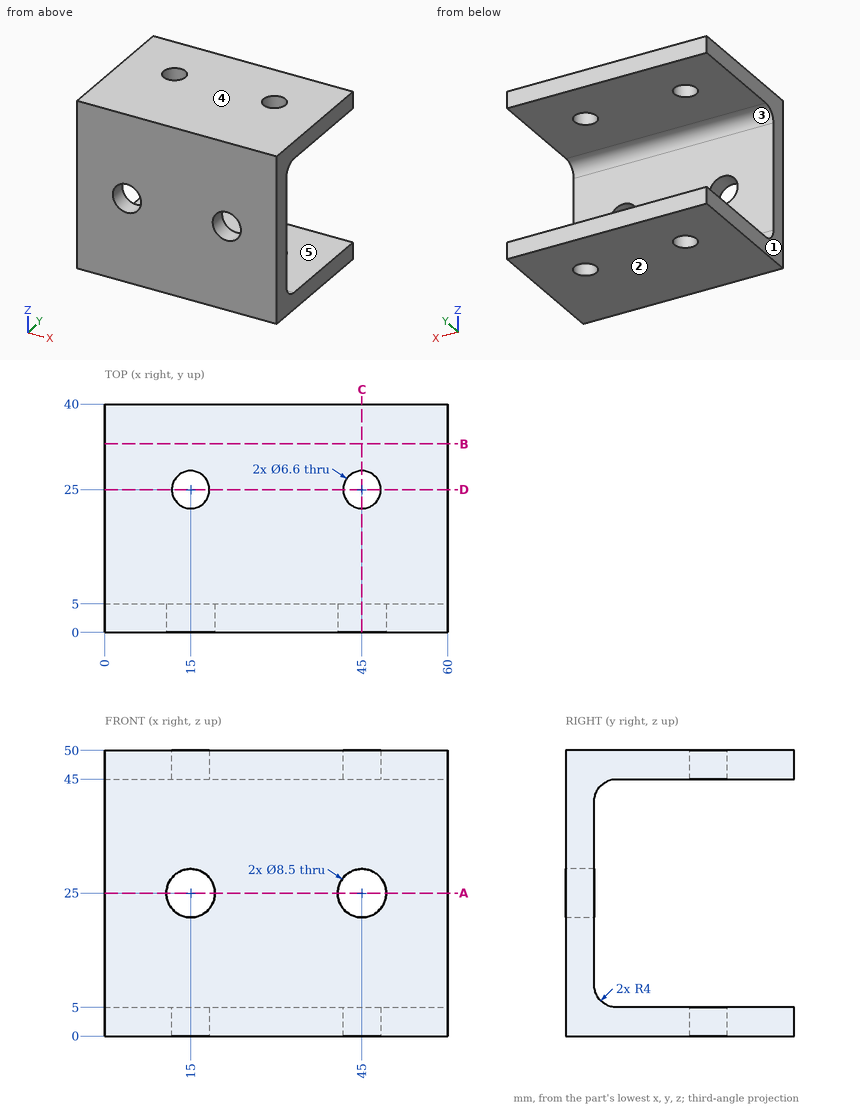
Here's the drawing with two shaded views (mm, measured from the low corner). I have some questions. A direction names the side the tool comes from. Give positions to 0.01 mm unless a question says otherwise; leave off trailing zeros. Order: outer loops, then holes, each group sorted by start corner. A loop starts at its lowest first (then second) coordinate and runs counter-clockwise, first axis right, second up. Notation, with made-up numbers: (70, 66.25) -> (109, 66.25) arc R19 ccw to (109, 90.25) -> close; hole circle Ø8 at (19, 22). An arc over 180 degrees is marked (long way). One line per item, written item: value. Start each with the question number.
1. Will these pins go through, and if not, where does the flat tip stop? pin 1 Ø1 at (x, y) = (51.5, 24) entering from -Z; pin 2 Ø1 at (x, z) = (47, 18) entering from +Y.
2. Imagine slicing it at D-D, the plane y = 25. List the corners of the cut face in (x, z) for me, plus the area to 3 significant figures.
3. Imagine slicing it at A-A, the plane z = 25. List the corners of the cut face in (x, y) for me.
4. Imagine slicing it at C-C, the plane x = 45. List the corners of the cut face in (y, z) for me, plus the area to 3 significant figures.
5. I need wall thicknesses on probe 1 along X at (y, z) = (1, 25); probe 2 along Z at (x, y) = (52.5, 24); probe 3 along Y at (x, z) = (15, 3). Which ranges of each line are inside material? Lowest first, please. Write a range as from..to.
6. Imagine slicing it at B-B, the plane y = 33. List the corners of the cut face in (x, z) for me, plus the area to 3 significant figures.
7. We'd pull the mould along Z, two halves only. Please class the marked faces 1, 2 and 3: released by +Z, released by -Z, zero draft, split by the parting line, or undercut.
8. For the marked faces 4 and 5, which set-ups out of +Z, -Z, +X, -X, +Y, -Y let a thin tool reach every point of the face, with its end or its side?
Values follow:
1. pin 1: stops at z = 0
1. pin 2: stops at y = 5
2. outline: (0, 0) -> (11.7, 0) -> (11.7, 5) -> (0, 5) -> close; (0, 45) -> (11.7, 45) -> (11.7, 50) -> (0, 50) -> close; (18.3, 0) -> (41.7, 0) -> (41.7, 5) -> (18.3, 5) -> close; (18.3, 45) -> (41.7, 45) -> (41.7, 50) -> (18.3, 50) -> close; (48.3, 0) -> (60, 0) -> (60, 5) -> (48.3, 5) -> close; (48.3, 45) -> (60, 45) -> (60, 50) -> (48.3, 50) -> close
2. area: 468 mm2
3. outline: (0, 0) -> (10.75, 0) -> (10.75, 5) -> (0, 5) -> close; (19.25, 0) -> (40.75, 0) -> (40.75, 5) -> (19.25, 5) -> close; (49.25, 0) -> (60, 0) -> (60, 5) -> (49.25, 5) -> close
4. outline: (0, 0) -> (21.7, 0) -> (21.7, 5) -> (9, 5) arc R4 cw to (5, 9) -> (5, 20.75) -> (0, 20.75) -> close; (0, 29.25) -> (5, 29.25) -> (5, 41) arc R4 cw to (9, 45) -> (21.7, 45) -> (21.7, 50) -> (0, 50) -> close; (28.3, 0) -> (40, 0) -> (40, 5) -> (28.3, 5) -> close; (28.3, 45) -> (40, 45) -> (40, 50) -> (28.3, 50) -> close
4. area: 498 mm2
5. probe 1: x = 0..10.75, 19.25..40.75, 49.25..60
5. probe 2: z = 0..5, 45..50
5. probe 3: y = 0..21.7, 28.3..40
6. outline: (0, 0) -> (60, 0) -> (60, 5) -> (0, 5) -> close; (0, 45) -> (60, 45) -> (60, 50) -> (0, 50) -> close
6. area: 600 mm2
7. face 1: zero draft
7. face 2: released by -Z
7. face 3: undercut
8. face 4: +Z, +X, -X, +Y, -Y
8. face 5: +X, -X, +Y
